Autodesk Fusion 360 part; units mm, degrees
sketch "Sketch1" plane through (0, 0, 0) normal (0, 1, 0) x (1, 0, 0)
  line L0 (0, 0) -> (24, 0)
  line L1 (0, 0) -> (0, -24)
  circle A0 centre (6, -6) radius 2.8
  line L2 (0, -24) -> (24, 0)
  line L3 (0, 0) -> (12, 0)
  line L4 (12, 0) -> (12, -12)
  line L5 (12, -12) -> (0, -12)
  line L6 (0, -12) -> (0, 0)
  line L7 (3, 0) -> (3, -23)
  line L8 (3, -3) -> (21, -3)
  dimension "d3" = 5.6
  dimension "d4" = 6
  dimension "d5" = 6
  dimension "d6" = 12
  dimension "d7" = 12
  dimension "d14" = 3
  dimension "d15" = 3
extrude "Extrude1" add sketch "Sketch1" along normal blind 17 contours L0 L1 L3 L5 L6 L7 | L0 L3 L4 L7 L8 | L4 L5 L7 L8
extrude "Extrude2" add sketch "Sketch1" along normal blind 2 contours L1 L2 L5 L7 | L0 L2 L4 L8 | L2 L5 L7 | L2 L4 L8
extrude "Extrude3" add sketch "Sketch1" along normal blind 17 contours L1 L2 L5 L7 | L0 L2 L4 L8
extrude "Extrude4" add sketch "Sketch1" against normal blind 2 from surface at 17 contours L2 L5 L7 | L2 L4 L8
sketch "Sketch2" plane through (0, 0, 3) normal (0, 0, 1) x (1, 0, 0)
  line L0 (21, 15) -> (12, 15)
  line L1 (12, 15) -> (12, 2)
  line L2 (12, 2) -> (21, 2)
  line L3 (21, 2) -> (21, 15)
  line L4 (12, 10) -> (21, 10) construction
  circle A0 centre (16.5, 10) radius 2.25
  point P0 (12, 10)
  point P1 (12, 8.5)
  dimension "d21" = 1.5
  dimension "d22" = 4.5
extrude "Extrude5" cut sketch "Sketch2" against normal through all contours A0
sketch "Sketch3" plane through (3, 0, 0) normal (1, 0, 0) x (0, 0, -1)
  line L0 (-12, 15) -> (-21, 15)
  line L1 (-21, 15) -> (-21, 2)
  line L2 (-21, 2) -> (-12, 2)
  line L3 (-12, 2) -> (-12, 15)
  line L4 (-12, 10) -> (-21, 10) construction
  circle A0 centre (-16.5, 10) radius 2.25
  point P0 (-12, 8.5)
  point P1 (-12, 10)
  dimension "d25" = 1.5
  dimension "d26" = 4.5
extrude "Extrude6" cut sketch "Sketch3" against normal through all contours A0
equation "d8 = 20 mm - 3 mm"
Check sheet for the modelled part. Datum: model origin and axes. Units: mm. A direction names the side the tool comes from. Coordinates: 2 decimals unless noted, no trailing zeros. Write each loop counter-clockwise with the first axis right and the second up, starting at its lowest first coordinate (ties: lowest second). Pieces come first, ordered by that corner, then holes. Notation, with made-up numbers: M 43,83.25 L 101,83.25 A20 cw 101,109.25 Z; hole C -35,9.25 d2. An arc over 180 degrees is marked long. Use one line per item in the form item = value.
Item 1: Gauge pin test, flat ends, axial feed: pin 1 Ø7 at (x, z) = (7.5, 17) entering from +Y; pin 2 Ø2 at (x, y) = (13.5, 11) entering from +Z; pin 3 Ø1.5 at (y, z) = (5.5, 14) entering from +X; pin 4 Ø7 at (x, y) = (8, 7.5) entering from +Z. Record the tip position at first contact, or that the pin passes through.
Answer below:
pin_1 = 17
pin_2 = 3
pin_3 = 3
pin_4 = 12
Item 2: Sectioned sample at B-B, the plane x = 6. Record the cut outline in (y, z), and give its area (3 significant figures).
Answer below:
outline = M 0,0 L 17,0 L 17,3.2 L 0,3.2 Z; M 0,8.8 L 17,8.8 L 17,18 L 15,18 L 15,12 L 2,12 L 2,18 L 0,18 Z
area = 133 mm^2
Item 3: Set-up check for faces 5 (the face through (8, 8, 12)), 6 (the face through (12, 1, 12)): record each of +Z, -Z, +X, -X, +Y, -Y from which the full face is reachable in a straight line by a thin tool's end or side.
Answer below:
face_5 = +Z, +X
face_6 = +Z, +X, +Y, -Y
Item 4: Release check for a two-part mould opening along Y. For faces 1 (the face through (9, 17, 9)), 2 (the face through (12, 8, 0)), 3 (the face through (15, 2, 6)), 4 (the face through (3, 7, 16)) record: pulls with the +Y half, pulls with the -Y half, needs draft (parallel to the pull), parting line crosses it, or undercut.
Answer below:
face_1 = pulls with the +Y half
face_2 = needs draft
face_3 = undercut
face_4 = undercut
Item 5: Sectioned sample at D-D, the plane x = 2. Record the cut outline in (y, z).
Answer below:
outline = M 0,0 L 17,0 L 17,22 L 0,22 Z; hole C 10,16.5 d4.5
Item 6: Sectioned sample at A-A, the plane y = 10. Record the cut outline in (x, z).
Answer below:
outline = M 0,0 L 14.25,0 L 14.25,3 L 12,3 L 12,12 L 3,12 L 3,14.25 L 0,14.25 Z; M 0,18.75 L 3,18.75 L 3,21 L 0,24 Z; M 18.75,0 L 24,0 L 21,3 L 18.75,3 Z; hole C 6,6 d5.6
Item 7: Sectioned sample at C-C, the plane z = 6. Record the cut outline in (x, y), and give its area (3 significant figures).
Answer below:
outline = M 0,0 L 3.2,0 L 3.2,17 L 0,17 Z; M 8.8,0 L 18,0 L 18,2 L 12,2 L 12,15 L 18,15 L 18,17 L 8.8,17 Z
area = 133 mm^2
Item 8: Material ranges on L1, parallel to X at y = 8.25, z = 6; L2, parallel to Y at x = 19, z = 3.75; L3, parallel to Y at x = 16.5, z = 1.5, recorded low to high. Write a range as from..to.
Answer below:
L1 = 0..3.2, 8.8..12
L2 = 0..2, 15..17
L3 = 0..7.75, 12.25..17
